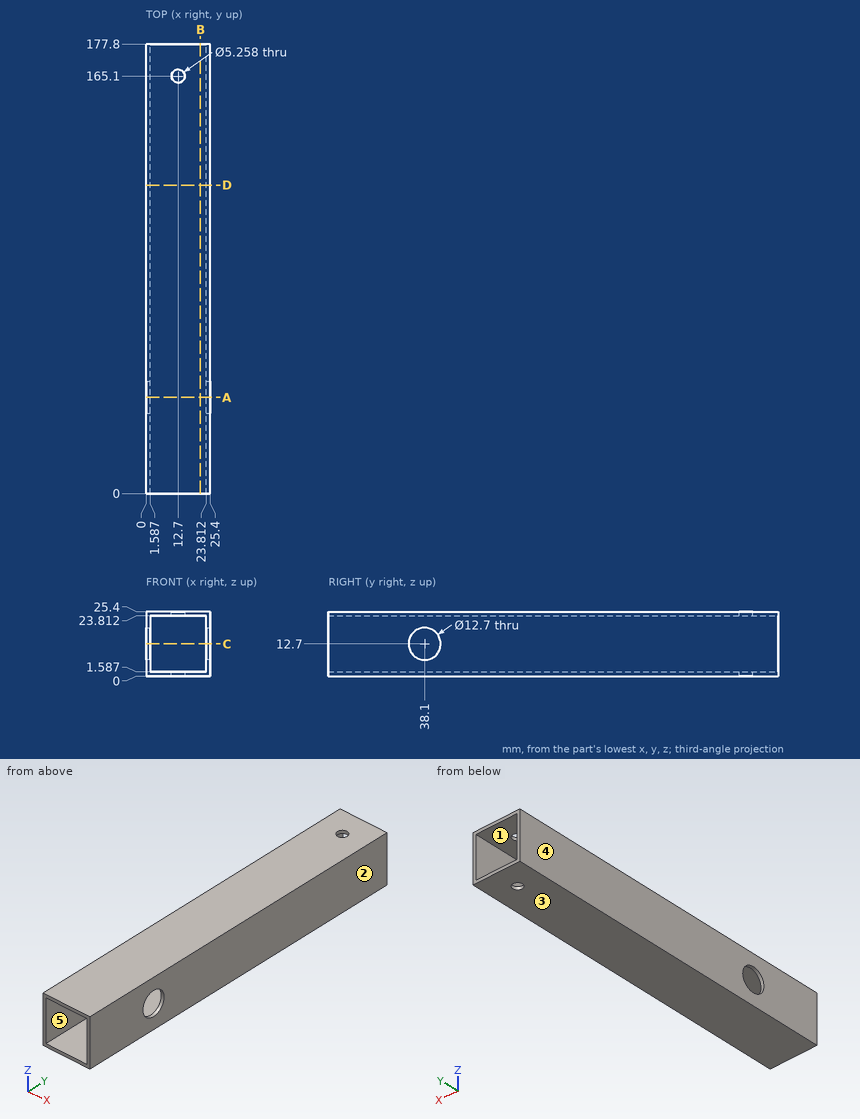
Geometry: see drawing. Coordinates: mm, zero at the bounding-box minimum. A direction names the side the tool comes from. Round coordinates to 2 decimals unless told otherwise and drop trailing zeros. Order: outer loops, then holes, each group sorted by start corner. A loop starts at its lowest first (then second) coordinate and runs counter-clockwise, first axis right, second up. Notation, with made-up numbers: (11, -3) -> (65, -3) arc R30 ccw to (65, 34) -> close; hole circle Ø7 at (63, 11). An arc over 180 degrees is marked (long way). Write each question's results on one line, items separated by ' | '.
Q1. Section query C-C (z = 12.7). Output: boundary loops of the cut face in (x, y).
Response values:
outline: (0, 0) -> (1.59, 0) -> (1.59, 31.75) -> (0, 31.75) -> close; (0, 44.45) -> (1.59, 44.45) -> (1.59, 177.8) -> (0, 177.8) -> close; (23.81, 0) -> (25.4, 0) -> (25.4, 31.75) -> (23.81, 31.75) -> close; (23.81, 44.45) -> (25.4, 44.45) -> (25.4, 177.8) -> (23.81, 177.8) -> close
Q2. Access query for the marked faces 4 and 5. Directions: +Z, -Z, +X, -X, +Y, -Y. A direction counts if a zero-diameter tool reaches every point of the face in a straight line with its end or side. Return the directions, or none.
Response values:
face 4: +Z, -Z, -X, +Y, -Y | face 5: +Y, -Y
Q3. Section query A-A (y = 38.1). Output: boundary loops of the cut face in (x, z).
Response values:
outline: (0, 0) -> (25.4, 0) -> (25.4, 6.35) -> (23.81, 6.35) -> (23.81, 1.59) -> (1.59, 1.59) -> (1.59, 6.35) -> (0, 6.35) -> close; (0, 19.05) -> (1.59, 19.05) -> (1.59, 23.81) -> (23.81, 23.81) -> (23.81, 19.05) -> (25.4, 19.05) -> (25.4, 25.4) -> (0, 25.4) -> close
Q4. Pull-direction query (X, two-part tool) for the marked faces 1, 2 and 3; classes: released by +X, released by -X, zero draft, split by the parting line, or undercut.
Response values:
face 1: undercut | face 2: released by +X | face 3: zero draft
Q5. Section query D-D (y = 122). Output: boundary loops of the cut face in (x, z), and give its area (3 significant figures).
Response values:
outline: (0, 0) -> (25.4, 0) -> (25.4, 25.4) -> (0, 25.4) -> close; hole (1.59, 1.59) -> (23.81, 1.59) -> (23.81, 23.81) -> (1.59, 23.81) -> close | area: 151 mm²
Q6. Section query B-B (x = 21.5). Output: boundary loops of the cut face in (y, z).
Response values:
outline: (0, 0) -> (177.8, 0) -> (177.8, 1.59) -> (0, 1.59) -> close; (0, 23.81) -> (177.8, 23.81) -> (177.8, 25.4) -> (0, 25.4) -> close
Q7. Ray query, line 1 along Z through (x, y) = (5.25, 68.5); line 2 along Y through (x, z) = (24.65, 12.7); line 3 along Y through (x, z) = (12.7, 25.05). Return the intervals inside material, ascending.
Response values:
line 1: 0 to 1.59, 23.81 to 25.4 | line 2: 0 to 31.75, 44.45 to 177.8 | line 3: 0 to 162.47, 167.73 to 177.8
